Read the model definition and answer for the solid it produces. Units are mm, in the model's axes. Face numbers are marked on the shaded views. Coordinates: 2 decimals unless noted, no trailing zeros. Write each loop counter-clockwise with the first axis right and the second up, starting at its lowest first coordinate (ties: lowest second). Pieces come first, ordered by that corner, then holes.
(1) Find the intervals of material crossed by probe 1 along Y at (x, z) = (6.25, 3.3); probe 2 along X at (y, z) = (153, 2.25); probe 3 along Y at (x, z) = (63.5, 3.3), in increasing order.
(2) Section B-B on x = -85.5 is taken. Write down the section's boundary in (y, z), then the cut area to 4 significant figures.
(3) The mould has two halves that part along X. Classify the marked faces 1 and 2: +X half, -X half, draft (parallel to the pull), parting line (faces both ways), or undercut.
(4) Section C-C on y = 87 is taken. Write down the section's boundary in (x, z).
(5) Given pin 1 (1.5 mm diameter, centred on x = 30, z = 5, fed in from -Y); pin 2 (6 mm diameter, centred on x = 20.5, y = 117, fed in from +Z); pin 3 (5 mm diameter, centred on x = -51.5, z = 5, fed in from +Y); pin 4 (0.6 mm diameter, centred on y = 189.5, z = 8, fed in from -X), each flat-ended and moving along its own axis, determine where each tip first touches the part or whether it passes through.
from build123d import *

# Parameters (mm, degrees)
SKETCH002_W            = 205
SKETCH002_H            = 115
PAD003_DEPTH           = 1.5
SKETCH003_W            = 205
SKETCH003_H            = 115
SKETCH003_W_2          = 200
SKETCH003_H_2          = 110
PAD002_DEPTH           = 3
SKETCH006_W            = 20
SKETCH006_H            = 1
PAD005_DEPTH           = 8.5
PAD006_DEPTH           = 10
PAD008_DEPTH           = 28.857143
LINEARPATTERN001_COUNT = 3
LINEARPATTERN001_PITCH = 58.714286
FILLET001_R            = 2
CHAMFER001_SIZE        = 1


with BuildPart() as part:
    # Sketch002 → Pad003 (new body)
    with BuildSketch(Plane.XY):
        Rectangle(SKETCH002_W, SKETCH002_H)
    extrude(amount=-PAD003_DEPTH)

    # Sketch003 → Pad002 (join)
    with BuildSketch(Plane.XY):
        Rectangle(SKETCH003_W, SKETCH003_H)
        Rectangle(SKETCH003_W_2, SKETCH003_H_2, mode=Mode.SUBTRACT)
    extrude(amount=PAD002_DEPTH)

    # Sketch006 → Pad005 (join)
    with BuildSketch(Plane.XY.offset(3)):
        with Locations((0, 57)):
            Rectangle(SKETCH006_W, SKETCH006_H)
    extrude(amount=PAD005_DEPTH)

    # Sketch007 → Pad006 (join, symmetric)
    with BuildSketch(Plane.YZ):
        Polygon((56.5, 11.5), (55.5, 10.5), (56.5, 9.5), align=None)
    extrude(amount=PAD006_DEPTH, both=True)

    # Sketch009 → Pad008 (join)
    with BuildSketch(Plane.YZ.offset(-73.142857)):
        with BuildLine():
            Line((-57.5, 3), (-57.8, 3.3))
            ThreePointArc((-57.8, 3.3), (-61.706992, 5.366488), (-61.216299, 0.973974))
            Line((-57.5, -0.49), (-61.216299, 0.973974))
            Line((-57.5, 3), (-57.5, -0.49))
        make_face()
        with BuildLine():
            Line((-61.183875, 4.183892), (-60.3, 5.067767))
            Line((-60.3, 5.067767), (-59.416106, 4.183873))
            ThreePointArc((-61.183875, 4.183892), (-60.300013, 2.05), (-59.416106, 4.183873))
        make_face(mode=Mode.SUBTRACT)
    pad008 = extrude(amount=PAD008_DEPTH)

    # LinearPattern001: Pad008 ×3
    with Locations(*[(i * LINEARPATTERN001_PITCH, 0, 0) for i in range(1, LINEARPATTERN001_COUNT)]):
        add(pad008)

    # Fillet001
    fillet001_edges = [part.edges().sort_by_distance(p)[0] for p in [
        (102.5, -57.5, 0.75),
        (102.5, 57.5, 0.75),
        (-102.5, 57.5, 0.75),
        (-102.5, -57.5, 0.75),
    ]]
    fillet(fillet001_edges, radius=FILLET001_R)

    # Chamfer001
    chamfer001_edges = [part.edges().sort_by_distance(p)[0] for p in [
        (0, 57.5, -1.5),
        (-101.914214, 56.914214, -1.5),
        (101.914214, 56.914214, -1.5),
        (-102.5, 0, -1.5),
        (102.5, 0, -1.5),
        (-101.914214, -56.914214, -1.5),
        (101.914214, -56.914214, -1.5),
        (0, -57.5, -1.5),
    ]]
    chamfer(chamfer001_edges, length=CHAMFER001_SIZE)


with BuildPart() as part_1:
    # Body001 placement: moved
    add(part.part.moved(Location((0, 133, 0))))


solid = part_1.part
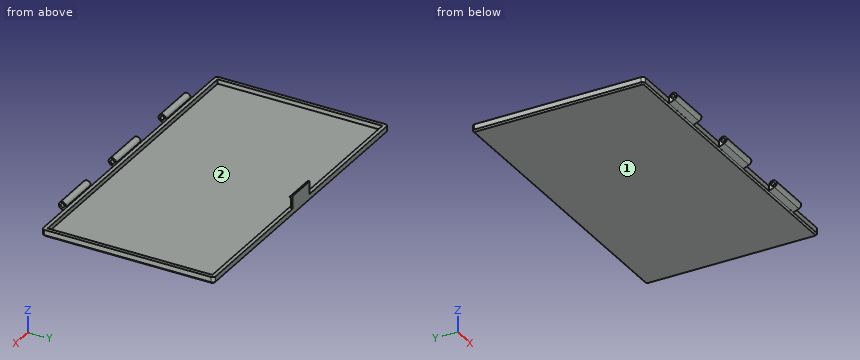
Response:
1. probe 1: y = 70.2 to 71.45, 73.95 to 75.2, 189.5 to 190.5
1. probe 2: x = -102.5 to -100, 100 to 102.5
1. probe 3: y = 70.2 to 71.45, 73.95 to 75.2
2. outline: (75.5, -0.5) - (76.5, -1.5) - (189.5, -1.5) - (190.5, -0.5) - (190.5, 3) - (188, 3) - (188, 0) - (78, 0) - (78, 3) - (75.5, 3) - close
2. area: 186.5 mm2
3. face 1: draft
3. face 2: undercut
4. outline: (-102.5, -0.5) - (-101.5, -1.5) - (101.5, -1.5) - (102.5, -0.5) - (102.5, 3) - (100, 3) - (100, 0) - (-100, 0) - (-100, 3) - (-102.5, 3) - close
5. pin 1: passes through
5. pin 2: stops at z = 0
5. pin 3: stops at y = 190.5
5. pin 4: stops at x = -10
